from build123d import *

# Parameters (mm, degrees)
F1_DEPTH = 270
F2_W     = 88
F2_H     = 212
F3_DEPTH = 178
F4_W     = 68
F4_H     = 172
F5_DEPTH = 5
F7_DEPTH = 146
F8_W     = 41
F8_H     = 340
F8_W_2   = 180.688232
F8_H_2   = 48.886035
F8_W_3   = 50.645926
F8_H_3   = 463.54628
F9_DEPTH = 200


with BuildPart() as f1:
    # F0 (on Front) → F1 (new body)
    with BuildSketch(Plane.XZ):
        with BuildLine():
            Line((-20, 505), (-665, 505))
            ThreePointArc((-665, 505), (-679.142136, 499.142136), (-685, 485))
            Line((-685, 485), (-685, 20))
            ThreePointArc((-685, 20), (-679.142136, 5.857864), (-665, 0))
            Line((-665, 0), (-20, 0))
            ThreePointArc((-20, 0), (-5.857864, 5.857864), (0, 20))
            Line((0, 20), (0, 485))
            ThreePointArc((0, 485), (-5.857864, 499.142136), (-20, 505))
        make_face()
    extrude(amount=-F1_DEPTH)

    # F2 (on face) → F3 (cut)
    with BuildSketch(Plane.XZ):
        with Locations((-541.250854, 134)):
            Rectangle(F2_W, F2_H)
        with Locations((-541.250854, 376)):
            Rectangle(F2_W, F2_H)
        with Locations((-423.250854, 134)):
            Rectangle(F2_W, F2_H)
        with Locations((-423.250854, 376)):
            Rectangle(F2_W, F2_H)
        with Locations((-305.250854, 134)):
            Rectangle(F2_W, F2_H)
        with Locations((-305.250854, 376)):
            Rectangle(F2_W, F2_H)
    extrude(amount=-F3_DEPTH, mode=Mode.SUBTRACT)

    # F4 (on face) → F5 (cut)
    with BuildSketch(Plane.XZ.offset(-178)):
        with Locations((-541.250854, 376)):
            Rectangle(F4_W, F4_H)
        with Locations((-423.250854, 376)):
            Rectangle(F4_W, F4_H)
        with Locations((-305.250854, 376)):
            Rectangle(F4_W, F4_H)
        with Locations((-305.250854, 134)):
            Rectangle(F4_W, F4_H)
        with Locations((-423.250854, 134)):
            Rectangle(F4_W, F4_H)
        with Locations((-541.250854, 134)):
            Rectangle(F4_W, F4_H)
    extrude(amount=-F5_DEPTH, mode=Mode.SUBTRACT)

    # F6 (on face) → F7 (cut)
    with BuildSketch(Plane.XZ):
        Polygon((-231.250854, 482), (-231.250854, 383), (-177.250854, 383), (-177.250854, 413), (-197.250854, 413), (-197.250854, 482), align=None)
        Polygon((-231.250854, 353), (-231.250854, 254), (-177.250854, 254), (-177.250854, 284), (-197.250854, 284), (-197.250854, 353), align=None)
        Polygon((-231.250854, 224), (-231.250854, 125), (-177.250854, 125), (-177.250854, 155), (-197.250854, 155), (-197.250854, 224), align=None)
        Polygon((-147.250854, 482), (-147.250854, 383), (-93.250854, 383), (-93.250854, 413), (-113.250854, 413), (-113.250854, 482), align=None)
        Polygon((-147.250854, 353), (-147.250854, 254), (-93.250854, 254), (-93.250854, 284), (-113.250854, 284), (-113.250854, 353), align=None)
        Polygon((-147.250854, 224), (-147.250854, 125), (-93.250854, 125), (-93.250854, 155), (-113.250854, 155), (-113.250854, 224), align=None)
    extrude(amount=-F7_DEPTH, mode=Mode.SUBTRACT)

    # F8 (on face) → F9 (cut)
    with BuildSketch(Plane.XZ):
        with Locations((-50.5, 295)):
            Rectangle(F8_W, F8_H)
        with Locations((-119.728997, 65.844511)):
            Rectangle(F8_W_2, F8_H_2)
        with Locations((-639.677037, 253.22686)):
            Rectangle(F8_W_3, F8_H_3)
    extrude(amount=-F9_DEPTH, mode=Mode.SUBTRACT)


solid = f1.part
Source: CAD feature listing. Evaluate the final solid. Frame: model axes, mm. Round coordinates to 2 decimals unless told otherwise and drop trailing zeros. Write each loop counter-clockwise with the first axis right and the second up, starting at its lowest first coordinate (ties: lowest second). Pieces come first, ordered by that corner, then holes. Notation, with made-up numbers: (39, -27) - (86, -27) arc R31 ccw to (86, 6) - close; hole circle Ø11 at (46, 13.25). An arc over 180 degrees is marked (long way). Use CSV: the item, a comma, the result in double quotes. Start each with the question number.
(1) First-contact query: pin 1 Ø20.5 at (x, z) = (-289, 403.5) entering from -Y. Flat tip, straight axial feed; report the tip coordinate or a pass-through.
(2) Cut plane C-C, the plane y = 168. Give the number of separate pieces and of enclosed holes in the cut face, and give its area (3 significant figures).
(3) Material intervals for probe 1 along X at (y, z) = (105.5, 80); probe 2 along Z at (x, y) = (-305, 97); probe 3 along X at (y, z) = (190.5, 453), sorted ascending. Write a range as [from, to].
(4) Cut plane B-B, the plane x = -307.5. Return loops of the section in (y, z).
(5) Mould query, pull axis Z, two halves, no side actions, for faces 1 (the face through (-231.251, 72, 304)), 2 (the face through (0, 133, 249)). Classes: pulls with the +Z half, pulls with the -Z half, needs draft (parallel to the pull), parting line crosses it, or undercut.
Geometry says:
1,pin 1,"y = 183"
2,separate pieces,"1"
2,enclosed holes,"9"
2,area,"187,000 mm²"
3,probe 1,"[-685, -665], [-614.35, -585.25], [-497.25, -467.25], [-379.25, -349.25], [-261.25, -210.07], [-29.38, 0]"
3,probe 2,"[0, 28], [240, 270], [482, 505]"
3,probe 3,"[-685, -665], [-614.35, -71], [-30, 0]"
4,outline,"(0, 0) - (270, 0) - (270, 505) - (0, 505) - (0, 482) - (178, 482) - (178, 462) - (183, 462) - (183, 290) - (178, 290) - (178, 270) - (0, 270) - (0, 240) - (178, 240) - (178, 220) - (183, 220) - (183, 48) - (178, 48) - (178, 28) - (0, 28) - close"
5,face 1,"undercut"
5,face 2,"needs draft"
